Autodesk Inventor part; units mm, degrees
ref_plane "YZ Plane" through (0, 0, 0) normal (1, 0, 0) x (0, 1, 0)
ref_plane "XZ Plane" through (0, 0, 0) normal (0, 1, 0) x (-1, 0, 0)
ref_plane "XY Plane" through (0, 0, 0) normal (0, 0, 1) x (1, 0, 0)
sketch "Sketch1" plane through (0, 0, 0) normal (0, 1, 0) x (-1, 0, 0)
  line L0 (0, 0) -> (-30, 0)
  line L1 (-30, 0) -> (-30, -20)
  line L2 (-30, -20) -> (0, -20)
  line L3 (0, -20) -> (0, 0)
  line L4 (0, 0) -> (-5, 0)
  line L5 (-15, -20) -> (0, -20)
  line L6 (0, -20) -> (0, 0)
  line L7 (-5, 0) -> (-5, -20)
  point P0 (-5, -20)
  dimension "d1" = 20
  dimension "d7" = 5
  dimension "d8" = 25
extrude "Extrusion1" add sketch "Sketch1" along normal blind 30 contours L3 L2 L7 L0
extrude "Extrusion3" add sketch "Sketch1" along normal blind 5 contours L7 L2 L1 L0
sketch "Sketch2" plane through (0, 5, 0) normal (0, 1, 0) x (1, 0, 0)
  line L0 (5, 0) -> (5, 20)
  line L1 (5, 0) -> (30, 0)
  point P0 (0, 0)
  point P1 (25, 10)
  dimension "d18" = 20
  dimension "d21" = 10
hole "Hole1" at (25, 5, -10) direction (0, -1, 0) diameter 3 end through all
sketch "Sketch3" plane through (5, 30, 0) normal (1, 0, 0) x (0, 0, -1)
  line L0 (20, -25) -> (20, 0)
  line L1 (0, 0) -> (20, 0)
  line L2 (0, -25) -> (20, -25)
  point P0 (0, -30)
  point P1 (10, -5)
  point P2 (20, -12.5)
  dimension "d30" = 10
  dimension "d32" = 20
hole "Hole2" at (5, 25, -10) direction (-1, 0, 0) diameter 3 end through all
properties part number "Fastener" material "ABS Plastic"
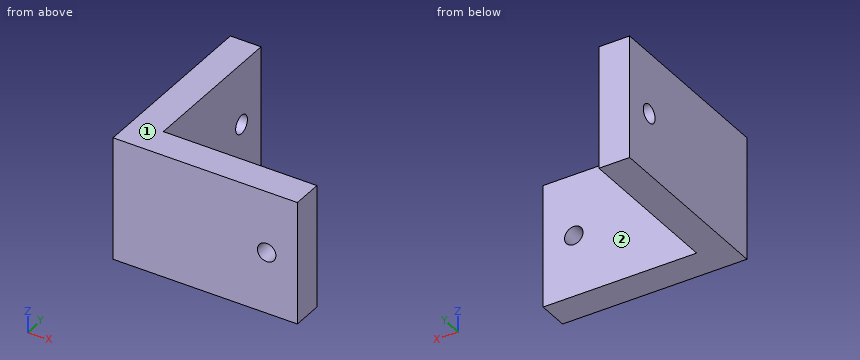
Geometry: final body of the model. Coordinates: model frame, mm. Face numbers are marked on the shaded views. A direction names the side the tool comes from. Round coordinates to 2 decimals unless told otherwise and drop trailing zeros. Order: outer loops, then holes, each group sorted by start corner. A loop starts at its lowest first (then second) coordinate and runs counter-clockwise, first axis right, second up. Notation, with made-up numbers: M 80.25,86 L 92.25,86 A26 ccw 92.25,109 Z; hole C 16,45.5 d9. An arc over 180 degrees is marked long. Use one line per item in the form item = value. Start each with the question number.
Q1. Access query for the marked faces 1 and 2. Directions: +Z, -Z, +X, -X, +Y, -Y. A direction counts if a zero-diameter tool reaches every point of the face in a straight line with its end or side. Return the directions, or none.
Q2. Pin query (flat end, axial travel): pin 1 Ø10 at (y, z) = (19, -6) entering from +X; pin 2 Ø5 at (x, z) = (5.5, -10.5) entering from -Y; pin 3 Ø4 at (x, z) = (25, -10) entering from +Y; pin 4 Ø1.5 at (x, y) = (6.5, 13) entering from +Z. Return the tip coordinate at first contact, or that it passes through.
Q3. Material intervals for line 1 (Y direction, x = 1.5, z = -10); line 2 (Z direction, x = 4.05, y = 25); line 3 (X direction, y = 25.5, z = -3.25), sorted ascending. Write a range as [from, to].
Q4. Cut plane D-D (z = -17.25). Return loops of the section in (x, y).
Q5. Cut plane A-A (y = 25). Return loops of the section in (x, z), and give its area (3 significant figures).
Q6. Cut plane B-B (z = -10). Return loops of the section in (x, y), and give its area (3 significant figures).
Geometry results:
q1.face_1 = +Z, +X, -X, +Y, -Y
q1.face_2 = +Z, -Z, +X, +Y
q2.pin_1 = 5
q2.pin_2 = 0
q2.pin_3 = 5
q2.pin_4 = through
q3.line_1 = [0, 23.5], [26.5, 30]
q3.line_2 = [-20, -11.5], [-8.5, 0]
q3.line_3 = [0, 5]
q4.outline = M 0,0 L 30,0 L 30,5 L 5,5 L 5,30 L 0,30 Z
q5.outline = M 0,-20 L 5,-20 L 5,-11.5 L 0,-11.5 Z; M 0,-8.5 L 5,-8.5 L 5,0 L 0,0 Z
q5.area = 85.0 mm^2
q6.outline = M 0,0 L 23.5,0 L 23.5,5 L 5,5 L 5,23.5 L 0,23.5 Z; M 0,26.5 L 5,26.5 L 5,30 L 0,30 Z; M 26.5,0 L 30,0 L 30,5 L 26.5,5 Z
q6.area = 245 mm^2
